Here's how the part is built. I have some questions about the finished solid (model axes, mm). A direction names the side the tool comes from. Give positions to 0.01 mm unless a question says otherwise; leave off trailing zeros. Answer in a Markdown table with one row per item. Add a question column.
Item 1: For P1, Ø2, axis at x = 2, y = 17.5, coming from the +Z side; P2, Ø8, axis at x = -37, z = -56, coming from the +Y side (3 decimals); P3, Ø4, axis at x = -36, y = -7.5, coming from the -Z side, each with a flat end and sliding along its axis, tell me the tip position at first contact or that it passes through.
Item 2: We'd pull the mould along Z, two halves only. Please class faces 1 (the face through (-2, 22.86, 67)), 2 (the face through (-2.6, 22.7, 46.2)), 3 (the face through (-34.64, 14.31, 58.78)): released by +Z, released by -Z, zero draft, split by the parting line, or undercut.
Item 3: Which directions (+Z, -Z, +X, -X, +Y, -Y) give clear straight access to the entire face, cutting with the end or side of a thin tool? Please do faces 4 (the face through (-33, -6, 12.573)), 5 (the face through (-40.04, 14.31, -54.76)), 6 (the face through (-11.483, 7.826, 6.452)).
Item 4: If we section it at A-A (y = -5): Give the number of separate pieces and of enclosed holes in the cut face, then the cut area to 3 significant figures.
Item 5: If I drill on line 1 (X direction, y = 19.5, z = 82.55); line 2 (Y direction, x = 22, z = 27) (3 decimals); line 3 (Z direction, x = 16.5, y = 12) (3 decimals), over which ranges is the centre line in solid material (lowest first)?
```python
from build123d import *

# Parameters (mm, degrees)
SKETCH1_W               = 86.36
SKETCH1_H               = 133.35
BOSS_EXTRUDE1_DEPTH     = 15.875
SKETCH2_W               = 86.36
SKETCH2_H               = 25.146
BOSS_EXTRUDE2_DEPTH     = 12.7
SKETCH5_R               = 1.7
SKETCH5_R_2             = 6
BOSS_EXTRUDE3_DEPTH     = 3.81
SKETCH6_R               = 19.685
CUT_EXTRUDE1_DEPTH      = 19.05
CHAMFER2_SIZE           = 0.508
SKETCH5_4_R             = 1.7
SKETCH5_4_R_2           = 6
BOSS_EXTRUDE4_DEPTH     = 6.35
CHAMFER1_SIZE           = 1.905
SKETCH7_R               = 5.08
CUT_EXTRUDE2_DEPTH      = 6.35
CUT_EXTRUDE3_DEPTH      = 3.175
CUT_EXTRUDE4_DEPTH      = 115.033341725
CUT_EXTRUDE4_DEPTH_BACK = 115.033341725
SKETCH8_3_R             = 2.2225
CUT_EXTRUDE5_DEPTH      = 115.033341725
CUT_EXTRUDE5_DEPTH_BACK = 115.033341725
SKETCH10_R              = 6.985
CUT_EXTRUDE6_DEPTH      = 12.7
CUT_EXTRUDE6_DEPTH_BACK = 12.7
SKETCH11_R              = 3.175
CHAMFER3_SIZE           = 26.416
CHAMFER4_SIZE           = 10.414
SKETCH13_R              = 19.05
CUT_EXTRUDE7_DEPTH      = 12.7
CHAMFER5_SIZE           = 1.27


with BuildPart() as part:
    # Sketch1 → Boss-Extrude1 (new body)
    with BuildSketch(Plane(origin=(0, 0, 0), x_dir=(1, 0, 0), z_dir=(0, 1, 0))):
        Rectangle(SKETCH1_W, SKETCH1_H)
    extrude(amount=BOSS_EXTRUDE1_DEPTH)

    # Sketch2 → Boss-Extrude2 (add)
    with BuildSketch(Plane.XZ):
        Rectangle(SKETCH2_W, SKETCH2_H)
    extrude(amount=BOSS_EXTRUDE2_DEPTH)

    # Sketch6 → Cut-Extrude1 (cut)
    with BuildSketch(Plane.XZ):
        with Locations((-2.032, 82.55)):
            Circle(SKETCH6_R)
    extrude(amount=-CUT_EXTRUDE1_DEPTH, mode=Mode.SUBTRACT)



with BuildPart() as body_2:
    # Sketch5 → Boss-Extrude3 (new body)
    with BuildSketch(Plane(origin=(0, 19.05, 0), x_dir=(-1, 0, 0), z_dir=(0, -1, 0))):
        with BuildLine():
            Line((-32.693781238, -66.874218762), (-17.018, -82.55))
            ThreePointArc((-17.018, -82.55), (2.032, -101.6), (21.082, -82.55))
            Line((21.082, -82.55), (36.757781238, -66.874218762))
            ThreePointArc((36.757781238, -66.874218762), (2.032, -44.45), (-32.693781238, -66.874218762))
        make_face()
        with Locations(Location((9.782, -69.126606241, 0), (0, 0, 90))):
            Circle(SKETCH5_R, mode=Mode.SUBTRACT)
        with Locations(Location((-5.718, -69.126606241, 0), (0, 0, 90))):
            Circle(SKETCH5_R, mode=Mode.SUBTRACT)
        with Locations(Location((-13.468, -82.55, 0), (0, 0, 90))):
            Circle(SKETCH5_R, mode=Mode.SUBTRACT)
        with Locations(Location((-5.718, -95.973393759, 0), (0, 0, 90))):
            Circle(SKETCH5_R, mode=Mode.SUBTRACT)
        with Locations(Location((9.782, -95.973393759, 0), (0, 0, 90))):
            Circle(SKETCH5_R, mode=Mode.SUBTRACT)
        with Locations(Location((17.532, -82.55, 0), (0, 0, 90))):
            Circle(SKETCH5_R, mode=Mode.SUBTRACT)
        with Locations(Location((2.032, -82.55, 0), (0, 0, 90))):
            Circle(SKETCH5_R_2, mode=Mode.SUBTRACT)
    extrude(amount=-BOSS_EXTRUDE3_DEPTH)

    # Chamfer2
    chamfer2_edges = [body_2.edges().sort_by_distance(p)[0] for p in [
        (-9.782, 22.86, 70.826606241),
        (-17.532, 22.86, 84.25),
        (-9.782, 22.86, 97.673393759),
        (5.718, 22.86, 97.673393759),
        (13.468, 22.86, 84.25),
        (5.718, 22.86, 70.826606241),
        (-2.032, 22.86, 101.6),
        (-2.032, 22.86, 88.55),
    ]]
    chamfer(chamfer2_edges, length=CHAMFER2_SIZE)


with BuildPart() as part_1:
    add(part.part)

    add(body_2.part)  # Boss-Extrude4 merges body 2
    # Sketch5<4> → Boss-Extrude4 (add)
    with BuildSketch(Plane(origin=(0, 19.05, 0), x_dir=(-1, 0, 0), z_dir=(0, -1, 0))):
        with BuildLine():
            Line((-32.693781238, -66.874218762), (-17.018, -82.55))
            ThreePointArc((-17.018, -82.55), (2.032, -101.6), (21.082, -82.55))
            Line((21.082, -82.55), (36.757781238, -66.874218762))
            ThreePointArc((36.757781238, -66.874218762), (2.032, -44.45), (-32.693781238, -66.874218762))
        make_face()
        with Locations(Location((9.782, -69.126606241, 0), (0, 0, 90))):
            Circle(SKETCH5_4_R, mode=Mode.SUBTRACT)
        with Locations(Location((-5.718, -69.126606241, 0), (0, 0, 90))):
            Circle(SKETCH5_4_R, mode=Mode.SUBTRACT)
        with Locations(Location((-13.468, -82.55, 0), (0, 0, 90))):
            Circle(SKETCH5_4_R, mode=Mode.SUBTRACT)
        with Locations(Location((-5.718, -95.973393759, 0), (0, 0, 90))):
            Circle(SKETCH5_4_R, mode=Mode.SUBTRACT)
        with Locations(Location((9.782, -95.973393759, 0), (0, 0, 90))):
            Circle(SKETCH5_4_R, mode=Mode.SUBTRACT)
        with Locations(Location((17.532, -82.55, 0), (0, 0, 90))):
            Circle(SKETCH5_4_R, mode=Mode.SUBTRACT)
        with Locations(Location((2.032, -82.55, 0), (0, 0, 90))):
            Circle(SKETCH5_4_R_2, mode=Mode.SUBTRACT)
    extrude(amount=BOSS_EXTRUDE4_DEPTH)

    # Chamfer1
    chamfer1_edges = [part_1.edges().sort_by_distance(p)[0] for p in [
        (-2.032, 15.875, 44.45),
        (-2.032, 22.86, 44.45),
    ]]
    chamfer(chamfer1_edges, length=CHAMFER1_SIZE)

    # Sketch7 → Cut-Extrude2 (cut)
    with BuildSketch(Plane(origin=(0, 15.875, 0), x_dir=(1, 0, 0), z_dir=(0, 1, 0))):
        with Locations((-37.338, -56.769)):
            Circle(SKETCH7_R)
    extrude(amount=CUT_EXTRUDE2_DEPTH, mode=Mode.SUBTRACT)

    # Sketch8 → Cut-Extrude3 (cut)
    with BuildSketch(Plane(origin=(0, 15.875, 0), x_dir=(1, 0, 0), z_dir=(0, 1, 0))):
        Polygon((-35.046242541, -53.63053412), (-38.910112452, -53.215046881), (-41.201869911, -56.353512761), (-39.629757459, -59.90746588), (-35.765887548, -60.322953119), (-33.474130089, -57.184487239), align=None)
        Polygon((-35.765887548, 60.322953119), (-33.474130089, 57.184487239), (-35.046242541, 53.63053412), (-38.910112452, 53.215046881), (-41.201869911, 56.353512761), (-39.629757459, 59.90746588), align=None)
        Polygon((28.625855338, 0), (30.568927669, -3.3655), (34.455072331, -3.3655), (36.398144662, 0), (34.455072331, 3.3655), (30.568927669, 3.3655), align=None)
    extrude(amount=-CUT_EXTRUDE3_DEPTH, mode=Mode.SUBTRACT)

    # Sketch8<3> → Cut-Extrude4 (cut, two sides: drawn at the far end of the back side and taken through both)
    with BuildSketch(Plane(origin=(0, 15.875, 0), x_dir=(1, 0, 0), z_dir=(0, 1, 0)).offset(-CUT_EXTRUDE4_DEPTH_BACK)):
        with Locations(Location((-37.338, -56.769, 0), (0, 0, 270))):
            Circle(SKETCH8_3_R)
        with Locations(Location((-37.338, 56.769, 0), (0, 0, 270))):
            Circle(SKETCH8_3_R)
        with Locations(Location((32.512, 0, 0), (0, 0, 270))):
            Circle(SKETCH8_3_R)
    extrude(amount=CUT_EXTRUDE4_DEPTH + CUT_EXTRUDE4_DEPTH_BACK, mode=Mode.SUBTRACT)

    # Sketch10 → Cut-Extrude5 (cut, two sides: drawn at the far end of the back side and taken through both)
    with BuildSketch(Plane(origin=(0, 15.875, 0), x_dir=(1, 0, 0), z_dir=(0, 1, 0)).offset(-CUT_EXTRUDE5_DEPTH_BACK)):
        with Locations(Location((-8.807904265, 0, 0), (0, 0, 270))):
            Circle(SKETCH10_R)
    extrude(amount=CUT_EXTRUDE5_DEPTH + CUT_EXTRUDE5_DEPTH_BACK, mode=Mode.SUBTRACT)

    # Sketch11 → Cut-Extrude6 (cut, two sides: drawn at the far end of the back side and taken through both)
    with BuildSketch(Plane.XY.offset(-CUT_EXTRUDE6_DEPTH_BACK)):
        with Locations((-8.807000374, 15.875)):
            Circle(SKETCH11_R)
    extrude(amount=CUT_EXTRUDE6_DEPTH + CUT_EXTRUDE6_DEPTH_BACK, mode=Mode.SUBTRACT)

    # Chamfer3
    chamfer3_edges = [part_1.edges().sort_by_distance(p)[0] for p in [
        (43.18, 7.9375, -66.675),
    ]]
    chamfer(chamfer3_edges, length=CHAMFER3_SIZE)

    # Chamfer4
    # the kernel refuses this chamfer: 10.414 mm, written as the material it takes off along each edge
    with BuildSketch(Plane(origin=(43.18, -26.781506637, 66.675), x_dir=(0.02749587661058629, 0, -0.9996219169112966), z_dir=(0, 1, 0))) as chamfer4_piece_1:
        Polygon((CHAMFER4_SIZE * 0.999621916911, CHAMFER4_SIZE * 0.0274958766106), (-CHAMFER4_SIZE * 0.0274958766106, CHAMFER4_SIZE * 0.999621916911), (0, 0), align=None)
    extrude(amount=69.438013273, mode=Mode.SUBTRACT)

    # Sketch13 → Cut-Extrude7 (cut)
    with BuildSketch(Plane.XZ.offset(12.7)):
        with Locations((-8.807904265, 0)):
            Circle(SKETCH13_R)
    extrude(amount=-CUT_EXTRUDE7_DEPTH, mode=Mode.SUBTRACT)

    # Chamfer5
    chamfer5_edges = [part_1.edges().sort_by_distance(p)[0] for p in [
        (-40.966177014, 15.875, 66.675),
        (-43.18, 15.875, 0),
        (-13.208, 15.875, -66.675),
        (29.972, 15.875, -53.467),
        (43.18, 15.875, 8.001),
        (38.634041338, 15.875, 60.806958662),
    ]]
    chamfer(chamfer5_edges, length=CHAMFER5_SIZE)


solid = part_1.part
```
Recorded:
| question | item | result |
|---|---|---|
| 1 | P1 | stops at z = 101.36 |
| 1 | P2 | stops at y = 15.875 |
| 1 | P3 | stops at z = -12.57 |
| 2 | face 1 | zero draft |
| 2 | face 2 | released by -Z |
| 2 | face 3 | undercut |
| 3 | face 4 | +Z, +X, -X, -Y |
| 3 | face 5 | +Y |
| 3 | face 6 | +Y, -Y |
| 4 | separate pieces | 2 |
| 4 | enclosed holes | 1 |
| 4 | area | 1,270 mm^2 |
| 5 | line 1 | x = -21.08 to -19.23, -15.83 to -8.03, 3.97 to 11.77, 15.17 to 17.02 |
| 5 | line 2 | y = 0 to 15.875 |
| 5 | line 3 | z = -66.675 to 66.675 |
